Geometry: final body of the model. Coordinates: model frame, mm. Give positions to 0.01 mm unless a question says otherwise; leave off trailing zeros. Write each loop counter-clockwise with the first axis right and the second up, starting at its lowest first coordinate (ties: lowest second). Pieces come first, ordered by that corner, then holes. Notation, with made-up numbers: (-28, 59) -> (-22, 59) arc R18 ccw to (-22, 67) -> close; hole circle Ø4 at (59.5, -18). An arc over 180 degrees is marked (long way). Answer as a JSON object with one key per item and string values.
from build123d import *

# Parameters (mm, degrees)
F0_R     = 161.29
F1_DEPTH = 1289.304
F2_R     = 4.826
F3_DEPTH = 905.002
F8_DEPTH = 1323.34


with BuildPart() as f1:
    # F0 (on Front) → F1 (new body)
    with BuildSketch(Plane.XZ):
        Circle(F0_R)
    extrude(amount=F1_DEPTH)

    # F2 (on face) → F3 (cut)
    with BuildSketch(Plane(origin=(0, 0, 0), x_dir=(-1, 0, 0), z_dir=(0, 1, 0))):
        with Locations((0, 77.724)):
            Circle(F2_R)
    extrude(amount=-F3_DEPTH, mode=Mode.SUBTRACT)

    # F4 (on Right) → F5 (revolve, cut)
    with BuildSketch(Plane.YZ):
        Polygon((-1291.5896564596, 140.5679192197), (-1289.304, 136.271), (-879.3132141796, 78.6505527405), (-879.3132141796, 82.6262438935), (-1288.7560755015, 140.1696853866), align=None)
    revolve(axis=Axis((0, -1084.3086070898, 107.4607763703), (0, 0.9902680687, -0.139173101)), mode=Mode.SUBTRACT)

    # F7 (on face) → F8 (cut)
    with BuildSketch(Plane(origin=(0, 0, 0), x_dir=(-1, 0, 0), z_dir=(0, 1, 0))):
        Polygon((88.3945971727, 168.1389510632), (0, 174.1231227369), (0, -186.8681758642), (195.7223266363, -99.0545749664), (195.7223266363, 72.0693692565), align=None)
    extrude(amount=-F8_DEPTH, mode=Mode.SUBTRACT)

    # F6 (on Right) → F9 (revolve, cut)
    with BuildSketch(Plane.YZ):
        Polygon((36.6785619574, 104.2698238297), (36.2579483429, 109.0774594427), (-321.6055191638, 77.7684629458), (-321.1849055493, 72.9608273328), align=None)
    revolve(axis=Axis((0, -142.6737854104, 93.4229611943), (0, -0.9961946981, -0.0871557427)), mode=Mode.SUBTRACT)


solid = f1.part
Q1. Cut plane A-A (y = -787.5). Return the cut outline in (x, z).
Values:
{"outline": "(0, -161.29) arc R161.29 ccw to (0, 161.29) -> (0, 82.55) arc R4.83 cw to (0, 72.9) -> close"}
Q2. Cut plane B-B (x = 68). Return the cut outline in (y, z).
Values:
{"outline": "(-1289.3, -146.25) -> (0, -146.25) -> (0, 146.25) -> (-1289.3, 146.25) -> close"}
Q3. Material intervals for L1, parallel to X at y = -306, z = -141; L2, parallel to X at y = -100.5, z = -30; L3, parallel to Z at x = 77.5, y = -122.5, sorted ascending. Write a range as from..to.
Values:
{"L1": "0..78.32", "L2": "0..158.48", "L3": "-141.45..141.45"}
Q4. Mould query, pull axis Z, two halves, no side actions, for faces 1 (the cylindrical face through (161.25, -635.63, -3.55)), 2 (the flat face through (62, -1289.304, 2)), 3 (the cylindrical face through (4.825, -158.329, 91.947)). Classes: pulls with the +Z half, pulls with the -Z half, needs draft (parallel to the pull), parting line crosses it, or undercut.
Values:
{"face 1": "parting line crosses it", "face 2": "needs draft", "face 3": "undercut"}
Q5. First-contact query: P1, Ø12, axis at x = 40, y = -201, coming from the +Z side; P2, Ø8, axis at y = -545.5, z = -77, coming from the +X side; P3, Ø10, axis at x = 28, y = -197.5, coming from the -Z side. Flat tips, straight axial feed; report the tip coordinate or a pass-through.
Values:
{"P1": "z = 157.67", "P2": "x = 143.82", "P3": "z = -159.64"}
